Here's how the part is built. I have some questions about the finished solid (model axes, mm). A direction names the side the tool comes from. Round coordinates to 2 decimals unless told otherwise and drop trailing zeros. Order: outer loops, then holes, each group sorted by start corner. A loop starts at its lowest first (then second) coordinate and runs counter-clockwise, first axis right, second up. Notation, with made-up numbers: (85, 43) -> (125, 43) arc R34 cw to (125, 74) -> close; hole circle Ø8 at (35.25, -35). An arc over 180 degrees is marked (long way). One line per item, written item: value.
```python
from build123d import *

# Parameters (mm, degrees)
AUFSATZ_LINEAR_AUSTRAGEN1_DEPTH = 5
AUFSATZ_LINEAR_AUSTRAGEN2_DEPTH = 5
SCHNITT_LINEAR_AUSTRAGEN1_DEPTH = 384.76425055
SCHNITT_LINEAR_AUSTRAGEN2_DEPTH = 384.76425055
SKIZZE5_R                       = 1.6
SCHNITT_LINEAR_AUSTRAGEN3_DEPTH = 384.666521865
FASE1_SIZE                      = 2


with BuildPart() as part:
    # Skizze1 → Aufsatz-Linear austragen1 (new body)
    with BuildSketch(Plane(origin=(0, 0, 0), x_dir=(1, 0, 0), z_dir=(0, 1, 0))):
        with BuildLine():
            Line((0, 0), (290, 0))
            ThreePointArc((290, 0), (251.147367097, 145), (145, 251.147367097))
            Line((145, 251.147367097), (0, 0))
        make_face()
    extrude(amount=AUFSATZ_LINEAR_AUSTRAGEN1_DEPTH)

    # Skizze2 → Aufsatz-Linear austragen2 (add)
    with BuildSketch(Plane(origin=(0, 5, 0), x_dir=(1, 0, 0), z_dir=(0, 1, 0))):
        with BuildLine():
            Line((0, 0), (149.9, 0))
            ThreePointArc((149.9, 0), (129.817208027, 74.95), (74.95, 129.817208027))
            Line((74.95, 129.817208027), (0, 0))
        make_face()
    extrude(amount=AUFSATZ_LINEAR_AUSTRAGEN2_DEPTH)

    # Skizze3 → Schnitt-Linear austragen1 (cut, through all)
    with BuildSketch(Plane(origin=(0, 10, 0), x_dir=(1, 0, 0), z_dir=(0, 1, 0))):
        Polygon((26.2, 45.379731158), (94.633560231, 84.889865579), (120.833560231, 39.510134421), (52.4, 0), (0, 0), align=None)
    extrude(amount=-SCHNITT_LINEAR_AUSTRAGEN1_DEPTH, mode=Mode.SUBTRACT)

    # Skizze4 → Schnitt-Linear austragen2 (cut, through all)
    with BuildSketch(Plane(origin=(0, 10, 0), x_dir=(1, 0, 0), z_dir=(0, 1, 0))):
        with BuildLine():
            Line((100, 0), (0, 0))
            Line((0, 0), (50, 86.602540378))
            ThreePointArc((50, 86.602540378), (86.602540378, 50), (100, 0))
        make_face()
    extrude(amount=-SCHNITT_LINEAR_AUSTRAGEN2_DEPTH, mode=Mode.SUBTRACT)

    # Skizze5 → Schnitt-Linear austragen3 (cut, through all)
    with BuildSketch(Plane(origin=(0, 5, 0), x_dir=(1, 0, 0), z_dir=(0, 1, 0))):
        with Locations(Location((95.879925069, 124.953151096, 0), (0, 0, 270))):
            Circle(SKIZZE5_R)
        with Locations(Location((224.122318632, 171.975103695, 0), (0, 0, 270))):
            Circle(SKIZZE5_R)
        with Locations(Location((145.511026371, 60.272640598, 0), (0, 0, 270))):
            Circle(SKIZZE5_R)
        with Locations(Location((280.083173338, 36.873649302, 0), (0, 0, 270))):
            Circle(SKIZZE5_R)
    extrude(amount=-SCHNITT_LINEAR_AUSTRAGEN3_DEPTH, mode=Mode.SUBTRACT)

    # Fase1
    fase1_edges = [part.edges().sort_by_distance(p)[0] for p in [
        (95.879925069, 0, -126.553151096),
        (224.122318632, 0, -173.575103695),
        (145.511026371, 0, -61.872640598),
        (280.083173338, 0, -38.473649302),
    ]]
    chamfer(fase1_edges, length=FASE1_SIZE)


solid = part.part
```
Q1. Which directions (+Z, -Z, +X, -X, +Y, -Y) give clear straight access to the entire face, cutting with the end or side of a thin tool? Please do faces 4 (the face through (173, 4, 0)), 5 (the face through (107.55, 5.07, -62.52)), 6 (the face through (108.92, 5.07, -32.63)), 7 (the face through (99.142, 5.07, -13.069)), 8 (the face through (130.36, 7.46, -74)).
Answers:
face 4: +Z, +X, -X, +Y, -Y
face 5: +Y, -Y
face 6: -X, +Y, -Y
face 7: +Z, -X, +Y, -Y
face 8: -Z, +X, +Y
Q2. For P1, Ø2, axis at x = 243.5, y = 4, coming from the -Z side; P2, Ø6, axis at y = 6.5, z = -95, coming from the -X side; P3, Ø2, axis at x = 109, y = 8, coming from the -Z side, each with a flat end and sliding along its axis, tell me the tip position at first contact or that it passes through.
Answers:
P1: z = -159.04
P2: x = 53.12
P3: z = -103.95
Q3. If we mould it in two halves opening along X, with no side actions, what happens to faces 1 (the face through (110, 10, -66)), 2 (the face through (82.39, 5.07, -77.82)), 3 (the face through (60.602, 5.07, -79.545))? For each: pulls with the +X half, pulls with the -X half, needs draft (parallel to the pull), parting line crosses it, or undercut.
Answers:
face 1: needs draft
face 2: undercut
face 3: pulls with the -X half
Q4. I want a section at C-C on x = 135.5. Write out the boundary of the cut face in (y, z).
Answers:
outline: (0, -234.69) -> (5, -234.69) -> (5, -64.11) -> (10, -64.11) -> (10, 0) -> (0, 0) -> close
Q5. I want a section at B-B on z = -47. Write out the boundary of the cut face in (x, y).
Answers:
outline: (116.51, 0) -> (286.17, 0) -> (286.17, 5) -> (142.34, 5) -> (142.34, 10) -> (116.51, 10) -> close
Q6. I want a section at D-D on z = -198.5. Write out the boundary of the cut face in (x, y).
Answers:
outline: (114.6, 0) -> (211.42, 0) -> (211.42, 5) -> (114.6, 5) -> close
Q7. I want a section at A-A on y = 7. Write out the boundary of the cut face in (x, z).
Answers:
outline: (50, -86.6) -> (74.95, -129.82) arc R149.9 ccw to (149.9, 0) -> (100, 0) arc R100 cw to (96.68, -25.56) -> (120.83, -39.51) -> (94.63, -84.89) -> (70.48, -70.94) arc R100 cw to start
Q8. I need wall thicknesses on line 1 along Y through (x, z) = (121.5, -127.5); line 2 along Z through (x, y) = (106.5, 7.75); line 3 along X through (y, z) = (3.75, -59). Which ranges of each line are inside material? Lowest first, please.
Answers:
line 1: 0 to 5
line 2: -105.49 to -64.34, -31.23 to 0
line 3: 109.58 to 144.54, 146.48 to 283.93
